Could you check a few things on this model? Use its own coordinates, in mm. Coordinates: 2 decimals unless noted, no trailing zeros. Write each loop counter-clockwise with the first axis right and the second up, starting at its lowest first coordinate (ties: lowest second). Pieces come first, ordered by that corner, then holes. Notation, with made-up numbers: M 23,53 L 81,53 A30 ccw 81,86 Z; hole C 37,78 d2. An arc over 180 degrees is marked long. Answer as CSV lines item,"result". Start each with the question number.
Item 1: Suppose I cut it at C-C, the plane x = 98.5. Write out the boundary of the cut face in (y, z).
Item 2: I'm going to push flat-ended pins straight in: P1, Ø1.5, axis at y = -10, z = 653, coming from the +X side (3 decimals); P2, Ø12, axis at y = -14, z = 492.5, coming from the -X side. Where does each tip first touch, or does it pass through?
Item 3: Suppose I cut it at B-B, the plane z = 566.5. Write out the boundary of the cut face in (x, y), and give its area (3 significant figures).
Item 4: If I drill on line 1 along X through (y, z) = (-10.5, 703); line 2 along X through (y, z) = (-8.75, 38.5), over which ranges is the centre line in solid material (lowest first)? Write a range as [from, to].
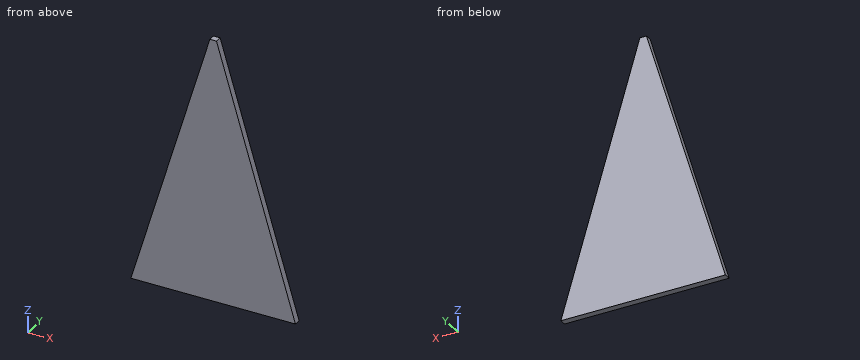
```python
from build123d import *

# Parameters (mm, degrees)
F2_W     = 500
F2_H     = 800
F3_DEPTH = 20
F4_SIZE2 = 799.99999
F4_SIZE  = 239.99999


# Not quite as in the source:
# - a fillet or chamfer is up to 0.001 mm smaller than in the source, because OpenCascade refuses the exact size


with BuildPart() as f3:
    # F2 (on Front) → F3 (new body)
    with BuildSketch(Plane.XZ):
        with Locations((0, 400)):
            Rectangle(F2_W, F2_H)
    extrude(amount=F3_DEPTH)

    # F4 (size 240 and 800 in the source; OpenCascade refuses exactly that, so slightly less here)
    f4_edges = [f3.edges().sort_by_distance(p)[0] for p in [
        (250, -10, 800),
        (-250, -10, 800),
    ]]
    f4_side = f3.faces().sort_by_distance((0, -10, 800))[0]
    chamfer(f4_edges, length=F4_SIZE, length2=F4_SIZE2, reference=f4_side)


solid = f3.part
```
Ans:
1,outline,"M -20,0 L 0,0 L 0,505 L -20,505 Z"
2,P1,"stops at x = 54.325"
2,P2,"stops at x = -104.05"
3,outline,"M -80.05,-20 L 80.05,-20 L 80.05,0 L -80.05,0 Z"
3,area,"3,200 mm^2"
4,line 1,"x = [-39.1, 39.1]"
4,line 2,"x = [-238.45, 238.45]"
